```python
from build123d import *

# Parameters (mm, degrees)
SKETCH1_R           = 37.5
BOSS_EXTRUDE1_DEPTH = 2
SKETCH5_R           = 28
BOSS_EXTRUDE5_DEPTH = 1
SKETCH2_R           = 24.9
BOSS_EXTRUDE2_DEPTH = 7
CHAMFER1_SIZE       = 1


with BuildPart() as part:
    # Sketch1 → Boss-Extrude1 (new body)
    with BuildSketch(Plane.XY):
        Circle(SKETCH1_R)
    extrude(amount=BOSS_EXTRUDE1_DEPTH)

    # Sketch5 → Boss-Extrude5 (add)
    with BuildSketch(Plane.XY.offset(2)):
        Circle(SKETCH5_R)
    extrude(amount=BOSS_EXTRUDE5_DEPTH)

    # Sketch2 → Boss-Extrude2 (add)
    with BuildSketch(Plane.XY.offset(3)):
        Circle(SKETCH2_R)
    extrude(amount=BOSS_EXTRUDE2_DEPTH)

    # Chamfer1
    chamfer1_edges = [part.edges().sort_by_distance(p)[0] for p in [
        (-28, 0, 3),
    ]]
    chamfer(chamfer1_edges, length=CHAMFER1_SIZE - 0.0001)  # a hair under: the kernel refuses the full size


solid = part.part
```
Work out the finished part from the listing and answer in its coordinate system (mm). A direction names the side the tool comes from. Coordinates: 2 decimals unless noted, no trailing zeros. Loops run counter-clockwise (first coordinate to the right, second up) from the corner with the lowest first, then second, coordinate; pieces in that order, holes last. Notation, with made-up numbers: (-30, 40.5) - (-7, 40.5) arc R23 ccw to (-7, 75.5) - close; hole circle Ø4 at (32.5, -25.75). An arc over 180 degrees is marked (long way). Use a Markdown table: item, result.
Item 1: The mould has two halves that part along Y. Classify faces 1 (the flat face through (-1, 1, 0)), 2 (the cylindrical face through (-4.88, 37.18, 0.99)): +Y half, -Y half, draft (parallel to the pull), parting line (faces both ways), or undercut.
Evaluation:
| item | result |
|---|---|
| face 1 | draft |
| face 2 | parting line |
Item 2: Find section C-C, the plane y = -32. Determine the outline of the cut face in (x, z), and give its area (3 significant figures).
Evaluation:
| item | result |
|---|---|
| outline | (-19.55, 0) - (19.55, 0) - (19.55, 2) - (-19.55, 2) - close |
| area | 78.2 mm2 |
Item 3: Find section D-D, the plane x = -31. Determine the outline of the cut face in (y, z), and give its area (3 significant figures).
Evaluation:
| item | result |
|---|---|
| outline | (-21.1, 0) - (21.1, 0) - (21.1, 2) - (-21.1, 2) - close |
| area | 84.4 mm2 |
Item 4: Find section B-B, the plane z = 5. Determine the outline of the cut face in (x, y), and give its area (3 significant figures).
Evaluation:
| item | result |
|---|---|
| outline | circle Ø49.8 at (0, 0) |
| area | 1,950 mm2 |
Item 5: Consider probe 1 along Z at (x, y) = (4.5, 30); probe 2 along Y at (x, z) = (13, 6.75); probe 3 along X at (y, z) = (10, 5). Determine where each line is inside the solid, lowest interval first. Write a range as from..to.
Evaluation:
| item | result |
|---|---|
| probe 1 | z = 0..2 |
| probe 2 | y = -21.24..21.24 |
| probe 3 | x = -22.8..22.8 |
Item 6: Given pin 1 Ø5 at (x, z) = (-28.5, 2.5) entering from -Y; pin 2 Ø1.5 at (x, y) = (-16, -21.5) entering from +Z, each flat-ended and moving along its own axis, determine where each tip first touches the part or whether it passes through.
Evaluation:
| item | result |
|---|---|
| pin 1 | stops at y = -26.97 |
| pin 2 | stops at z = 3 |
Item 7: For faces 3 (the flat face through (-28, -3, 2)), 4 (the flat face through (0, 0, 10)), determine the directions among +Z, -Z, +X, -X, +Y, -Y from which every point of the face is accessible in a straight line to the end or side of a thin tool.
Evaluation:
| item | result |
|---|---|
| face 3 | +Z |
| face 4 | +Z, +X, -X, +Y, -Y |
